Here's how the part is built. I have some questions about the finished solid (model axes, mm). Face numbers are marked on the shaded views. A direction names the side the tool comes from. Give positions to 0.01 mm unless a question says otherwise; leave off trailing zeros. Order: outer loops, then holes, each group sorted by start corner. A loop starts at its lowest first (then second) coordinate and runs counter-clockwise, first axis right, second up. Notation, with made-up numbers: (-36, -22.75) -> (-1, -22.75) arc R22 ccw to (-1, 14.25) -> close; hole circle Ø8 at (-14, 79.25). An arc over 180 degrees is marked (long way). Write each question's results on one line, items separated by ' | '. Start each with the question number.
Q1. Imagine slicing it at C-C, the plane z = 10. Please give me the cut outline in (x, y), then the cut area to 3 significant figures.
Q2. Imagine slicing it at A-A, the plane x = 0.5. Please give me the cut outline in (y, z).
Q3. I need wall thicknesses on line 1 along X through (y, z) = (-2.25, -14); line 2 along X through (y, z) = (-7.75, -4); line 3 along Z through (x, y) = (23, -3.5). Which ranges of each line are inside material? Lowest first, please. Write a range as [from, to].
Q4. Thinking about a two-plate mould opening in X: for the marked faces 1, 2 and 3, which applies, pulls with the +X half, pulls with the -X half, needs draft (parallel to the pull), parting line crosses it, or undercut?
Q5. Imagine slicing it at B-B, the plane y = -2.25. Please give me the cut outline in (x, z), then the cut area to 3 significant figures.
Q6. I'm going to push flat-ended pins straight in: pin 1 (25 mm diameter, centred on x = -4, z = 7.5, fed in from -Y); pin 2 (21 mm diameter, centred on x = -10, z = -7, fed in from +Y); pin 3 (2 mm diameter, centred on x = 5.5, y = -2, fed in from +Z). Where does each tip first touch, or does it pass through?
Q7. For the marked faces 4, 5 and 6, which set-ups out of +Z, -Z, +X, -X, +Y, -Y let a thin tool reach every point of the face, with its end or its side?
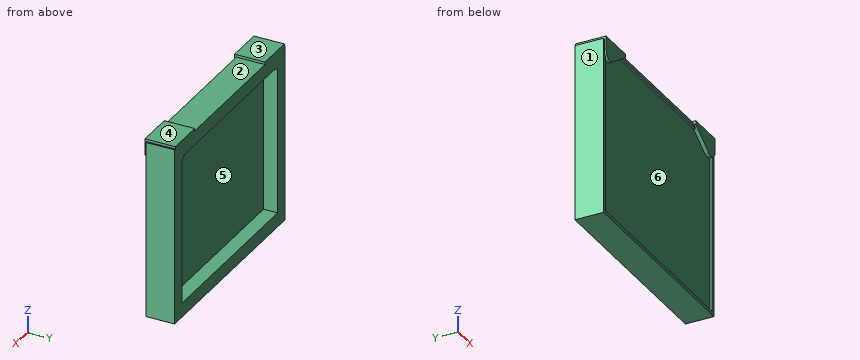
```python
from build123d import *

# Parameters (mm, degrees)
F0_W          = 59.5
F0_H          = 50.1
F1_DEPTH      = 8.1
F2_W          = 57.5
F2_H          = 48.1
F3_DEPTH      = 0.6
F4_W          = 51.5
F4_H          = 42.1
F5_DEPTH      = 4
F7_DEPTH      = 0.5
F7_DEPTH_BACK = 8.1


with BuildPart() as f1:
    # F0 (on Front) → F1 (new body)
    with BuildSketch(Plane.XZ):
        Rectangle(F0_W, F0_H)
    extrude(amount=F1_DEPTH)

    # F2 (on face) → F3 (cut)
    with BuildSketch(Plane.XZ.offset(8.1)):
        Rectangle(F2_W, F2_H)
    extrude(amount=-F3_DEPTH, mode=Mode.SUBTRACT)

    # F4 (on face) → F5 (cut)
    with BuildSketch(Plane(origin=(0, 0, 0), x_dir=(-1, 0, 0), z_dir=(0, 1, 0))):
        Rectangle(F4_W, F4_H)
    extrude(amount=-F5_DEPTH, mode=Mode.SUBTRACT)

    # F6 (on face) → F7 (join, two sides)
    with BuildSketch(Plane.XZ.offset(8.1)) as f7_sk:
        with BuildLine():
            ThreePointArc((25.93377, 20.016756), (28.190263, 19.911482), (29.35, 21.85))
            Line((29.35, 21.85), (29.35, 25.75))
            Line((29.35, 25.75), (18.95, 25.75))
            Line((18.95, 25.75), (18.95, 24.65))
            Line((18.95, 24.65), (25.93377, 20.016756))
        make_face()
        with BuildLine():
            Line((-18.95, 24.65), (-18.95, 25.75))
            Line((-18.95, 25.75), (-29.35, 25.75))
            Line((-29.35, 25.75), (-29.35, 21.85))
            ThreePointArc((-29.35, 21.85), (-28.190263, 19.911482), (-25.93377, 20.016756))
            Line((-25.93377, 20.016756), (-18.95, 24.65))
        make_face()
    extrude(amount=F7_DEPTH)
    extrude(f7_sk.sketch, amount=-F7_DEPTH_BACK)


solid = f1.part
```
Geometry check:
1) outline: (-29.75, -8.1) -> (-28.75, -8.1) -> (-28.75, -7.5) -> (28.75, -7.5) -> (28.75, -8.1) -> (29.75, -8.1) -> (29.75, 0) -> (25.75, 0) -> (25.75, -4) -> (-25.75, -4) -> (-25.75, 0) -> (-29.75, 0) -> close | area: 241 mm²
2) outline: (-8.1, -25.05) -> (0, -25.05) -> (0, -21.05) -> (-4, -21.05) -> (-4, 21.05) -> (0, 21.05) -> (0, 25.05) -> (-8.1, 25.05) -> (-8.1, 24.05) -> (-7.5, 24.05) -> (-7.5, -24.05) -> (-8.1, -24.05) -> close
3) line 1: [-29.75, -25.75], [25.75, 29.75] | line 2: [-29.75, -28.75], [28.75, 29.75] | line 3: [-25.05, -21.05], [21.05, 25.75]
4) face 1: pulls with the -X half | face 2: undercut | face 3: needs draft
5) outline: (-29.75, -25.05) -> (29.75, -25.05) -> (29.75, 25.05) -> (29.35, 25.05) -> (29.35, 25.75) -> (18.95, 25.75) -> (18.95, 25.05) -> (-18.95, 25.05) -> (-18.95, 25.75) -> (-29.35, 25.75) -> (-29.35, 25.05) -> (-29.75, 25.05) -> close; hole (-25.75, -21.05) -> (25.75, -21.05) -> (25.75, 20.14) -> (24.38, 21.05) -> (-24.38, 21.05) -> (-25.75, 20.14) -> close | area: 829 mm²
6) pin 1: y = -7.5 | pin 2: y = -4 | pin 3: z = 25.05
7) face 4: +Z, +X, -X, +Y, -Y | face 5: +Y | face 6: -Y
